Geometry: see drawing. Coordinates: mm, zero at the bounding-box minimum. A direction names the side the tool comes from. Round coordinates to 2 decimals unless told otherwise and drop trailing zeros. Loops run counter-clockwise (first coordinate to the right, second up) from the corner with the lowest first, then second, coordinate; pieces in that order, holes last. Notation, with made-up numbers: (-1, 18) - (58, 18) arc R24 cw to (58, 42) - close; hole circle Ø2 at (-24, 3). An arc over 180 degrees is marked (long way). Return JSON: item names as keys, results as strings. Group by question number.
1. Section A-A on x = 15. Return loops of the section in (y, z).
2. Section B-B on y = 21.5. Return loops of the section in (x, z), and give its area (3 significant figures).
3. Material intervals for probe 1 along Z at (x, y) = (27.7, 15); probe 2 along Y at (x, z) = (15, 6.5); probe 3 along X at (y, z) = (9.75, 9.75), sorted ascending.
4. Draft query along X for the marked faces 3, 4 and 5. Return one class per face: +X half, -X half, draft (parallel to the pull), parting line (faces both ways), or undercut.
5. Set-up query: the marked faces 1 and 2. Return all of +Z, -Z, +X, -X, +Y, -Y with unobstructed straight access to the full face (end or side cutting, diameter ignored); none if empty.
6. First-contact query: pin 1 Ø2.5 at (y, z) = (15, 12.5) entering from +X; pin 2 Ø4 at (y, z) = (24.5, 7.5) entering from -X; pin 3 Ø3.5 at (x, z) = (15.5, 17.5) entering from +Y; pin 4 Ø5 at (y, z) = (17, 19.5) entering from +X. Flat tips, straight axial feed; report the tip coordinate or a pass-through.
7. Section C-C on z = 21.5. Return loops of the section in (x, y) (1 decimal), and give its area (3 significant figures).
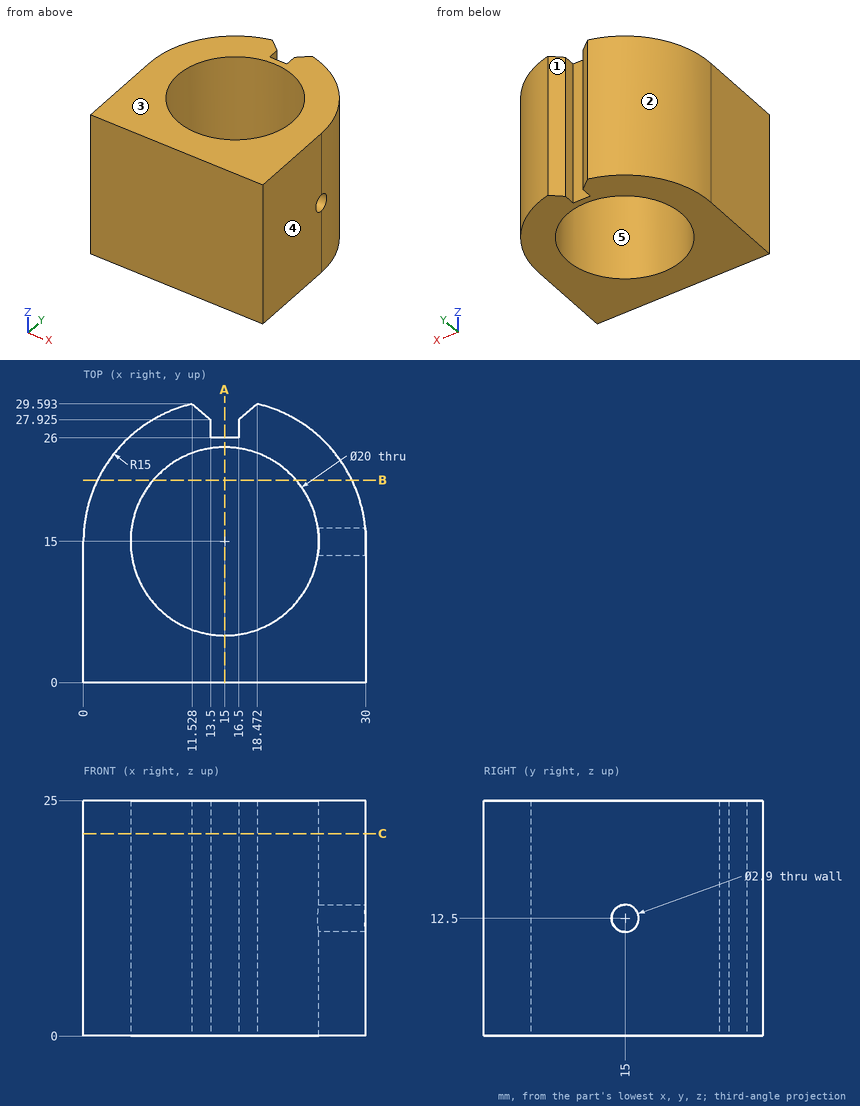
Taken from the geometry:
{
 "1": {"outline": "(0, 0) - (5, 0) - (5, 25) - (0, 25) - close; (25, 0) - (26, 0) - (26, 25) - (25, 25) - close"},
 "2": {"outline": "(1.48, 0) - (7.4, 0) - (7.4, 25) - (1.48, 25) - close; (22.6, 0) - (28.52, 0) - (28.52, 25) - (22.6, 25) - close", "area": "296 mm2"},
 "3": {"probe 1": "0 to 11.05, 13.95 to 25", "probe 2": "0 to 5, 25 to 26", "probe 3": "0 to 6.49, 23.51 to 30"},
 "4": {"face 3": "draft", "face 4": "+X half", "face 5": "undercut"},
 "5": {"face 1": "+Z, -Z, +Y", "face 2": "+Z, -Z, -X, +Y"},
 "6": {"pin 1": "x = 5.08", "pin 2": "x = 2.01", "pin 3": "y = 28.56", "pin 4": "x = 30"},
 "7": {"outline": "(0, 0) - (30, 0) - (30, 15) arc R15 ccw to (18.5, 29.6) - (16.5, 27.9) - (16.5, 26) - (13.5, 26) - (13.5, 27.9) - (11.5, 29.6) arc R15 ccw to (0, 15) - close; hole circle Ø20 at (15, 15)", "area": "473 mm2"}
}
